Model file for the job. Use its own axes, mm. Face numbers are marked on the shaded views. A direction names the side the tool comes from. Give positions to 0.01 mm unless a question says otherwise; leave off trailing zeros. Loops run counter-clockwise (first coordinate to the right, second up) from the corner with the lowest first, then second, coordinate; pieces in that order, holes last. Notation, with made-up numbers: (-26.75, 25) - (-8.75, 25) arc R28 cw to (-8.75, 60) - close; hole circle Ø1 at (67.5, 45). An arc over 180 degrees is marked (long way). Use a Markdown table: item, result.
from build123d import *

# Parameters (mm, degrees)
F1_DEPTH = 25.4


with BuildPart() as f1:
    # F0 (on Top) → F1 (new body)
    with BuildSketch(Plane.XY):
        Polygon((14.5529050286, 20.0303553717), (0, 64.8195915964), (-14.5529050286, 20.0303553717), align=None)
        Polygon((-14.5529050286, 20.0303553717), (-61.6470949714, 20.0303553717), (-23.5470949714, -7.6509149453), align=None)
        Polygon((-23.5470949714, -7.6509149453), (-38.1, -52.44015117), (0, -24.7588808529), align=None)
        Polygon((23.5470949714, -7.6509149453), (61.6470949714, 20.0303553717), (14.5529050286, 20.0303553717), align=None)
        Polygon((0, -24.7588808529), (38.1, -52.44015117), (23.5470949714, -7.6509149453), align=None)
        Polygon((14.5529050286, 20.0303553717), (-14.5529050286, 20.0303553717), (-23.5470949714, -7.6509149453), (0, -24.7588808529), (23.5470949714, -7.6509149453), align=None)
    extrude(amount=F1_DEPTH)


solid = f1.part
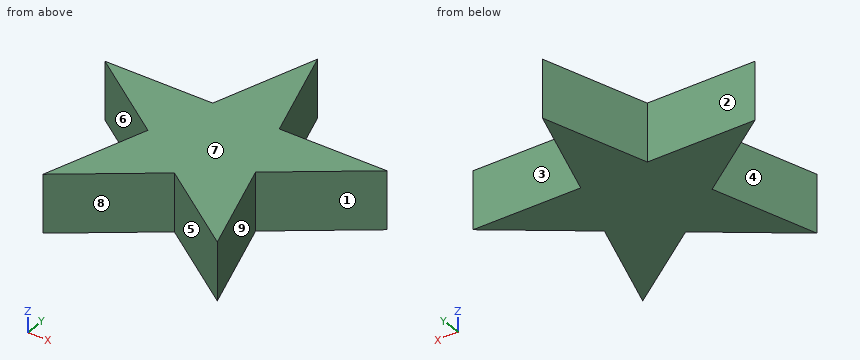
(1) Slice it at A-A, the plane z = 7.5. Write the cut outline in (x, y).
Computed:
| item | result |
|---|---|
| outline | (-61.65, 20.03) - (-23.55, -7.65) - (-38.1, -52.44) - (0, -24.76) - (38.1, -52.44) - (23.55, -7.65) - (61.65, 20.03) - (14.55, 20.03) - (0, 64.82) - (-14.55, 20.03) - close |
(2) Slice it at C-C, the plane x = 19. Write the cut outline in (y, z).
Computed:
| item | result |
|---|---|
| outline | (-38.56, 0) - (20.03, 0) - (20.03, 25.4) - (-38.56, 25.4) - close |
(3) Drill centre lines: probe 1 along X at (y, z) = (-45.5, 5.5) (3 decimals); probe 2 along X at (y, z) = (38, 11.25); probe 3 along X at (y, z) = (33, 19). Where is each one in solid material? Low to high. Write a range as [from, to].
Computed:
| item | result |
|---|---|
| probe 1 | [-35.845, -28.548], [28.548, 35.845] |
| probe 2 | [-8.71, 8.71] |
| probe 3 | [-10.34, 10.34] |
(4) Mould opens along Y. For the marked faces 6, 7, 8 and 9 say: pulls with the +Y half, pulls with the -Y half, needs draft (parallel to the pull), parting line crosses it, or undercut.
Computed:
| item | result |
|---|---|
| face 6 | undercut |
| face 7 | needs draft |
| face 8 | pulls with the -Y half |
| face 9 | undercut |
(5) Pin check, flat tips, straight feed: P1, Ø10, axis at y = 28.5, z = 17.5, coming from the +X side; P2, Ø5, axis at y = -19.5, z = 17.5, coming from the +X side; P3, Ø1.5, axis at y = -9, z = 16.5, coming from the +X side. Stop position of each tip, or through.
Computed:
| item | result |
|---|---|
| P1 | x = 13.43 |
| P2 | x = 28.21 |
| P3 | x = 24.23 |
(6) Slice it at B-B, the plane y = 29.5. Write the cut outline in (x, z).
Computed:
| item | result |
|---|---|
| outline | (-11.48, 0) - (11.48, 0) - (11.48, 25.4) - (-11.48, 25.4) - close |
(7) 3-axis set-ups, long thin cutter, end or side, ignore diameter. For the marked faces 1, 2, 3, 4 and 5: which of +Z, -Z, +X, -X, +Y, -Y reach the whole face in a straight line?
Computed:
| item | result |
|---|---|
| face 1 | +Z, -Z, +X |
| face 2 | +Z, -Z, -X, +Y |
| face 3 | +Z, -Z, +X, +Y |
| face 4 | +Z, -Z, -X |
| face 5 | +Z, -Z, -Y |
